```python
from build123d import *

# Parameters (mm, degrees)
F0_W     = 40
F0_H     = 40
F1_DEPTH = 25
F2_DEPTH = 40
F3_R     = 4.178344
F3_W     = 9.777684
F3_H     = 8.984899
F4_DEPTH = 40.001


with BuildPart() as f1:
    # F0 (on Top) → F1 (new body)
    with BuildSketch(Plane.XY):
        with Locations((-1.321308, 1.88122)):
            Rectangle(F0_W, F0_H)
    extrude(amount=F1_DEPTH)

    # F0 (on Top) → F2 (join)
    with BuildSketch(Plane.XY):
        with Locations((-1.321308, 1.88122)):
            Rectangle(F0_W, F0_H)
    extrude(amount=F2_DEPTH)

    # F3 (on face) → F4 (cut, through all)
    with BuildSketch(Plane.YZ.offset(18.678692)):
        with Locations((-9.117031, 31.843539)):
            Circle(F3_R)
        with Locations((12.420302, 28.143876)):
            Rectangle(F3_W, F3_H)
        Polygon((0, 16.252099), (-10.702601, 9.909815), (-3.831795, 5.417366), align=None)
    extrude(amount=-F4_DEPTH, mode=Mode.SUBTRACT)


solid = f1.part
```
Geometry: final body of the model. Coordinates: model frame, mm. A direction names the side the tool comes from. Round coordinates to 2 decimals unless told otherwise and drop trailing zeros. Order: outer loops, then holes, each group sorted by start corner. A loop starts at its lowest first (then second) coordinate and runs counter-clockwise, first axis right, second up. Notation, with made-up numbers: (-13, -10.75) -> (17, -10.75) arc R26 ccw to (17, 7.25) -> close; hole circle Ø9 at (-23, 43). An arc over 180 degrees is marked (long way). Use one line per item in the form item = value. Start each with the question number.
1. Cut plane B-B (z = 8.5). Return the cut outline in (x, y), then the cut area to 3 significant figures.
2. Reachability of faces 5 (the face through (-1, 12, 23.651)), 6 (the face through (-21.321, 2, 20)) from +Z, -Z, +X, -X, +Y, -Y: full face, straight path, thin tool, end or side. Return the list, or none.
3. Cut plane C-C (x = 10.5). Return the cut outline in (y, z).
4. Cut plane D-D (z = 30). Return the cut outline in (x, y).
5. Cut plane A-A (y = 14). Return the cut outline in (x, z), then the cut area to 3 significant figures.
6. Draft query along Y for faces 1 (the face through (-2, 21.881, 20)), 2 (the face through (-1.041, -5.276, 13.125)), 3 (the face through (-2, 2, 40)), 4 (the face through (-1.041, -1.943, 10.759)). Return one class per face: pulls with the +Y half, pulls with the -Y half, needs draft (parallel to the pull), parting line crosses it, or undercut.
7. Line query: probe 1 along Y at (x, z) = (-4.5, 24); probe 2 along Z at (x, y) = (-12, -5.5); probe 3 along Z at (x, y) = (0, 15). Output: solid intervals per line, ascending.
Solution:
q1.outline = (-21.32, -18.12) -> (18.68, -18.12) -> (18.68, -8.55) -> (-21.32, -8.55) -> close; (-21.32, -2.74) -> (18.68, -2.74) -> (18.68, 21.88) -> (-21.32, 21.88) -> close
q1.area = 1,370 mm^2
q2.face_5 = +X, -X
q2.face_6 = +Z, -Z, -X, +Y, -Y
q3.outline = (-18.12, 0) -> (21.88, 0) -> (21.88, 40) -> (-18.12, 40) -> close; hole circle Ø8.36 at (-9.12, 31.84); hole (-10.7, 9.91) -> (-3.83, 5.42) -> (0, 16.25) -> close; hole (7.53, 23.65) -> (17.31, 23.65) -> (17.31, 32.64) -> (7.53, 32.64) -> close
q4.outline = (-21.32, -18.12) -> (18.68, -18.12) -> (18.68, -12.87) -> (-21.32, -12.87) -> close; (-21.32, -5.37) -> (18.68, -5.37) -> (18.68, 7.53) -> (-21.32, 7.53) -> close; (-21.32, 17.31) -> (18.68, 17.31) -> (18.68, 21.88) -> (-21.32, 21.88) -> close
q5.outline = (-21.32, 0) -> (18.68, 0) -> (18.68, 23.65) -> (-21.32, 23.65) -> close; (-21.32, 32.64) -> (18.68, 32.64) -> (18.68, 40) -> (-21.32, 40) -> close
q5.area = 1,240 mm^2
q6.face_1 = pulls with the +Y half
q6.face_2 = undercut
q6.face_3 = needs draft
q6.face_4 = undercut
q7.probe_1 = -18.12 to 7.53, 17.31 to 21.88
q7.probe_2 = 0 to 6.51, 12.99 to 29.75, 33.94 to 40
q7.probe_3 = 0 to 23.65, 32.64 to 40
